Here's the drawing with two shaded views (mm, measured from the low corner). I have some questions. A direction names the side the tool comes from. Give positions to 0.01 mm unless a question says otherwise; leave off trailing zeros. Write each loop counter-clockwise with the first axis right and the second up, starting at its lowest first coordinate (ties: lowest second). Pieces come first, ordered by that corner, then holes. Notation, with made-up numbers: M 11.5,-36 L 67.5,-36 A14 cw 67.5,-25 Z; hole C 42,61.5 d8. An arc over 180 degrees is marked long. Use one line per item in the form item = value.
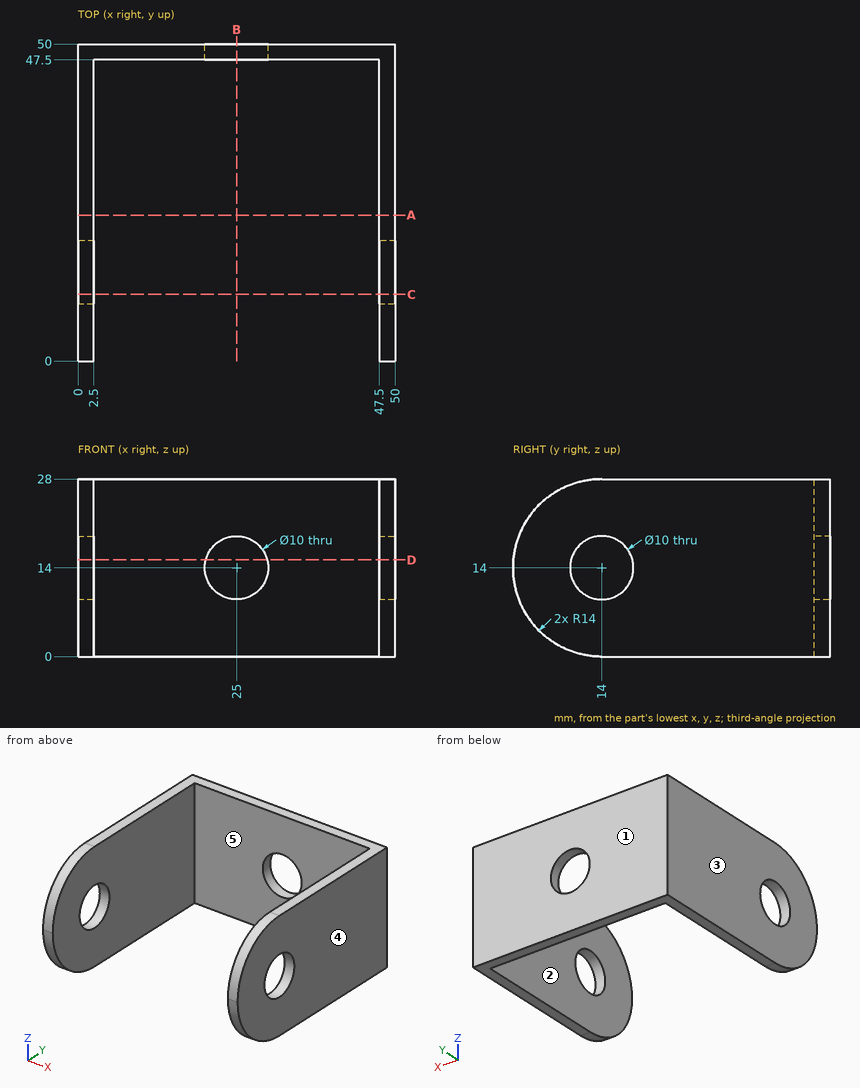
1) I want a section at A-A, the plane y = 23. Please give me the cut outline in (x, z), plus the area to 3 significant figures.
Checked values:
outline = M 0,0 L 2.5,0 L 2.5,28 L 0,28 Z; M 47.5,0 L 50,0 L 50,28 L 47.5,28 Z
area = 140 mm2
2) If I drill on L1, parallel to X at y = 49, z = 14; L2, parallel to Z at x = 1.7, y = 14; L3, parallel to X at y = 21, z = 23.5, over which ranges is the centre line in solid material (lowest first)?
Checked values:
L1 = 0 to 20, 30 to 50
L2 = 0 to 9, 19 to 28
L3 = 0 to 2.5, 47.5 to 50
3) I want a section at B-B, the plane x = 25. Please give me the cut outline in (y, z), plus the area to 3 significant figures.
Checked values:
outline = M 47.5,0 L 50,0 L 50,9 L 47.5,9 Z; M 47.5,19 L 50,19 L 50,28 L 47.5,28 Z
area = 45.0 mm2
4) For pin 1 Ø8 at (y, z) = (36, 18.5) entering from -X; pin 2 Ø6 at (y, z) = (14, 14) entering from -X; pin 3 Ø8 at (x, z) = (14.5, 13) entering from -Y, each with a flat end and sliding along its axis, tell me the tip position at first contact or that it passes through.
Checked values:
pin_1 = 0
pin_2 = through
pin_3 = 47.5
5) I want a section at C-C, the plane y = 10.5. Please give me the cut outline in (x, z).
Checked values:
outline = M 0,0.44 L 2.5,0.44 L 2.5,10.43 L 0,10.43 Z; M 0,17.57 L 2.5,17.57 L 2.5,27.56 L 0,27.56 Z; M 47.5,0.44 L 50,0.44 L 50,10.43 L 47.5,10.43 Z; M 47.5,17.57 L 50,17.57 L 50,27.56 L 47.5,27.56 Z
6) I want a section at D-D, the plane z = 15.25. Please give me the cut outline in (x, y), plus the area to 3 significant figures.
Checked values:
outline = M 0,0.06 L 2.5,0.06 L 2.5,9.16 L 0,9.16 Z; M 0,18.84 L 2.5,18.84 L 2.5,47.5 L 20.16,47.5 L 20.16,50 L 0,50 Z; M 29.84,47.5 L 47.5,47.5 L 47.5,18.84 L 50,18.84 L 50,50 L 29.84,50 Z; M 47.5,0.06 L 50,0.06 L 50,9.16 L 47.5,9.16 Z
area = 290 mm2
7) Thinking about a two-plate mould opening in X: for the marked faces 3, 4 and 5, which applies, released by +X, released by -X, zero draft, split by the parting line, or undercut?
Checked values:
face_3 = released by -X
face_4 = released by +X
face_5 = undercut
8) For the marked faces 1 and 2, which set-ups out of +Z, -Z, +X, -X, +Y, -Y let a thin tool reach every point of the face, with its end or its side?
Checked values:
face_1 = +Z, -Z, +X, -X, +Y
face_2 = +Z, -Z, -Y
